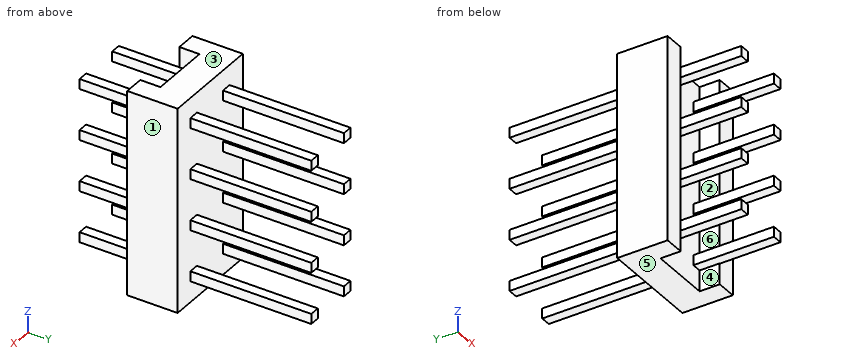
```python
from build123d import *

# Parameters (mm, degrees)
EXTRUDE_1_DEPTH        = 2.54
EXTRUDE_START          = -5.5
SKETCH_2_W             = 0.5
SKETCH_2_H             = 0.5
EXTRUDE_2_DEPTH        = 11.5
PATTERN_LINEAR_1_COUNT = 4
PATTERN_LINEAR_1_PITCH = 2.54


with BuildPart() as part:
    # Эскиз1 → Бобышка-Вытянуть1 (new body)
    with BuildSketch(Plane.XY):
        Polygon((-2.5, 0), (-2.5, 2.5), (2.5, 2.5), (2.5, 0), (1.5, 0), (1.5, 1), (-1.5, 1), (-1.5, 0), align=None)
    extrude_1 = extrude(amount=EXTRUDE_1_DEPTH)

    # Эскиз2 → Бобышка-Вытянуть2 (add)
    with BuildSketch(Plane(origin=(0, 2.5, 0), x_dir=(1, 0, 0), z_dir=(0, 1, 0)).offset(EXTRUDE_START)):
        with Locations((-1.236880281, -1.29)):
            Rectangle(SKETCH_2_W, SKETCH_2_H)
        with Locations((1.27, -1.29)):
            Rectangle(SKETCH_2_W, SKETCH_2_H)
    extrude_2 = extrude(amount=EXTRUDE_2_DEPTH)

    # Линейный массив1: Бобышка-Вытянуть1, Бобышка-Вытянуть2 ×4
    with Locations(*[(0, 0, -i * PATTERN_LINEAR_1_PITCH) for i in range(1, PATTERN_LINEAR_1_COUNT)]):
        add(extrude_1)
        add(extrude_2)


solid = part.part
```
Input: part model. Units: mm. Frame: model coordinates. Face numbers are marked on the shaded views. A direction names the side the tool comes from. Give positions to 0.01 mm unless a question says otherwise; leave off trailing zeros. Loops run counter-clockwise (first coordinate to the right, second up) from the corner with the lowest first, then second, coordinate; pieces in that order, holes last. Notation, with made-up numbers: M 5,-23.5 L 56,-23.5 A18 ccw 56,4.5 Z; hole C -31,22.5 d8. An arc over 180 degrees is marked long. Answer as CSV lines item,"result". Start each with the question number.
1. Pull-direction query (X, two-part tool) for the marked faces 1, 2 and 3; classes: released by +X, released by -X, zero draft, split by the parting line, or undercut.
2. Section B-B on z = 1.75. Return loops of the section in (x, y).
3. Line query: L1, parallel to Z at x = 1.05, y = -0.5; L2, parallel to X at y = 7.25, z = -6.25; L3, parallel to Y at x = -1.6, z = -7. Output: solid intervals per line, ascending.
4. Section C-C on x = -1.7. Return loops of the section in (y, z).
5. Pin query (flat end, axial travel): P1, Ø6, axis at y = 6, z = -4.5, coming from the +X side; P2, Ø1, axis at x = 0, z = -1, coming from the +Y side; P3, Ø0.6, axis at x = 1.5, y = 5.5, coming from the +Z side. Return the tip coordinate at first contact, or that it passes through.
6. Section A-A on y = 7.75. State how many separate pieces and enclosed holes the cut face has, plus the area to 3 significant figures.
7. Reachability of the marked faces 4, 5 and 6 from +Z, -Z, +X, -X, +Y, -Y: full face, straight path, thin tool, end or side. Return the list, or none.
8. Section D-D on x = -0.7. Return loops of the section in (y, z).
Computed values:
1,face 1,"released by +X"
1,face 2,"undercut"
1,face 3,"zero draft"
2,outline,"M -2.5,0 L -1.5,0 L -1.5,1 L 1.5,1 L 1.5,0 L 2.5,0 L 2.5,2.5 L -2.5,2.5 Z"
3,L1,"z = -6.58 to -6.08, -4.04 to -3.54, -1.5 to -1, 1.04 to 1.54"
3,L2,"x = -1.49 to -0.99, 1.02 to 1.52"
3,L3,"y = 0 to 2.5"
4,outline,"M 0,-7.62 L 2.5,-7.62 L 2.5,2.54 L 0,2.54 Z"
5,P1,"stops at x = 1.52"
5,P2,"stops at y = 2.5"
5,P3,"stops at z = 1.54"
6,separate pieces,"8"
6,enclosed holes,"0"
6,area,"2.00 mm²"
7,face 4,"-Z, -Y"
7,face 5,"-Z, +X, -X, +Y, -Y"
7,face 6,"-Y"
8,outline,"M 1,-7.62 L 2.5,-7.62 L 2.5,2.54 L 1,2.54 Z"
